```python
from build123d import *

# Parameters (mm, degrees)
SKETCH_1_W                         = 200
SKETCH_1_H                         = 27
SM_BASE_FLANGE_1_DEPTH             = 1
SM_EDGE_FLANGE_1_STRIP_W           = 7
SM_EDGE_FLANGE_1_STRIP_H           = 1
SM_EDGE_FLANGE_1_STRIP_CUT_DEPTH   = 200
SM_EDGE_FLANGE_1_STRIP_2_W         = 7
SM_EDGE_FLANGE_1_STRIP_2_H         = 1
SM_EDGE_FLANGE_1_STRIP_CUT_2_DEPTH = 200
SM_EDGE_FLANGE_1_DEPTH             = 200
SM_EDGE_FLANGE_1_BEND_DEPTH        = 200
SM_EDGE_FLANGE_2_STRIP_W           = 7
SM_EDGE_FLANGE_2_STRIP_H           = 1
SM_EDGE_FLANGE_2_STRIP_CUT_DEPTH   = 200
SM_EDGE_FLANGE_2_STRIP_2_W         = 7
SM_EDGE_FLANGE_2_STRIP_2_H         = 1
SM_EDGE_FLANGE_2_STRIP_CUT_2_DEPTH = 200
SM_EDGE_FLANGE_2_DEPTH             = 200
SM_EDGE_FLANGE_2_BEND_DEPTH        = 200
CUT_EXTRUDE_1_DEPTH                = 10
PATTERN_LINEAR_1_COUNT             = 5
PATTERN_LINEAR_1_PITCH             = 20
PATTERN_LINEAR_1_COL_COUNT         = 5
PATTERN_LINEAR_1_COL_PITCH         = 20


# Sheet-metal steps are written as plain solids
with BuildPart() as part:
    # Sketch 1 → 基体-法兰1 (new body)
    with BuildSketch(Plane.XY):
        Rectangle(SKETCH_1_W, SKETCH_1_H)
    extrude(amount=-SM_BASE_FLANGE_1_DEPTH)

    # 边线-法兰1 strip (across the edge) → 边线-法兰1 strip cut (cut)
    with BuildSketch(Plane(origin=(100, 13.5, 0), x_dir=(0, -1, 0), z_dir=(-1, 0, 0))):
        with Locations((-1, -0.5)):
            Rectangle(SM_EDGE_FLANGE_1_STRIP_W, SM_EDGE_FLANGE_1_STRIP_H)
    extrude(amount=SM_EDGE_FLANGE_1_STRIP_CUT_DEPTH, mode=Mode.SUBTRACT)

    # 边线-法兰1 strip 2 (across the edge) → 边线-法兰1 strip cut 2 (cut)
    with BuildSketch(Plane(origin=(-100, -13.5, 0), x_dir=(0, 1, 0), z_dir=(1, 0, 0))):
        with Locations((-1, -0.5)):
            Rectangle(SM_EDGE_FLANGE_1_STRIP_2_W, SM_EDGE_FLANGE_1_STRIP_2_H)
    extrude(amount=SM_EDGE_FLANGE_1_STRIP_CUT_2_DEPTH, mode=Mode.SUBTRACT)

    # 边线-法兰1 section (across the edge) → 边线-法兰1 (add)
    with BuildSketch(Plane(origin=(100, 13.5, 0), x_dir=(0, -1, 0), z_dir=(-1, 0, 0))):
        with BuildLine():
            Line((0, 1.5), (0, 6.5))
            Line((0, 6.5), (1, 6.5))
            Line((1, 6.5), (1, 1.5))
            ThreePointArc((1, 1.5), (1.439339828, 0.439339828), (2.5, 0))
            Line((2.5, 0), (2.5, -1))
            ThreePointArc((2.5, -1), (0.732233047, -0.267766953), (0, 1.5))
        make_face()
    extrude(amount=SM_EDGE_FLANGE_1_DEPTH)

    # 边线-法兰1 section 2 (across the edge) → 边线-法兰1 bend (add)
    with BuildSketch(Plane(origin=(-100, -13.5, 0), x_dir=(0, 1, 0), z_dir=(1, 0, 0))):
        with BuildLine():
            Line((0, 1.5), (0, 6.5))
            Line((0, 6.5), (1, 6.5))
            Line((1, 6.5), (1, 1.5))
            ThreePointArc((1, 1.5), (1.439339828, 0.439339828), (2.5, 0))
            Line((2.5, 0), (2.5, -1))
            ThreePointArc((2.5, -1), (0.732233047, -0.267766953), (0, 1.5))
        make_face()
    extrude(amount=SM_EDGE_FLANGE_1_BEND_DEPTH)

    # 边线-法兰2 strip (across the edge) → 边线-法兰2 strip cut (cut)
    with BuildSketch(Plane(origin=(-100, 13.5, 6.5), x_dir=(0, 0, -1), z_dir=(1, 0, 0))):
        with Locations((-1, -0.5)):
            Rectangle(SM_EDGE_FLANGE_2_STRIP_W, SM_EDGE_FLANGE_2_STRIP_H)
    extrude(amount=SM_EDGE_FLANGE_2_STRIP_CUT_DEPTH, mode=Mode.SUBTRACT)

    # 边线-法兰2 strip 2 (across the edge) → 边线-法兰2 strip cut 2 (cut)
    with BuildSketch(Plane(origin=(100, -13.5, 6.5), x_dir=(0, 0, -1), z_dir=(-1, 0, 0))):
        with Locations((-1, -0.5)):
            Rectangle(SM_EDGE_FLANGE_2_STRIP_2_W, SM_EDGE_FLANGE_2_STRIP_2_H)
    extrude(amount=SM_EDGE_FLANGE_2_STRIP_CUT_2_DEPTH, mode=Mode.SUBTRACT)

    # 边线-法兰2 section (across the edge) → 边线-法兰2 (add)
    with BuildSketch(Plane(origin=(-100, 13.5, 6.5), x_dir=(0, 0, -1), z_dir=(1, 0, 0))):
        with BuildLine():
            Line((0, 1.5), (0, 4))
            Line((0, 4), (1, 4))
            Line((1, 4), (1, 1.5))
            ThreePointArc((1, 1.5), (1.439339828, 0.439339828), (2.5, 0))
            Line((2.5, 0), (2.5, -1))
            ThreePointArc((2.5, -1), (0.732233047, -0.267766953), (0, 1.5))
        make_face()
    extrude(amount=SM_EDGE_FLANGE_2_DEPTH)

    # 边线-法兰2 section 2 (across the edge) → 边线-法兰2 bend (add)
    with BuildSketch(Plane(origin=(100, -13.5, 6.5), x_dir=(0, 0, -1), z_dir=(-1, 0, 0))):
        with BuildLine():
            Line((0, 1.5), (0, 4))
            Line((0, 4), (1, 4))
            Line((1, 4), (1, 1.5))
            ThreePointArc((1, 1.5), (1.439339828, 0.439339828), (2.5, 0))
            Line((2.5, 0), (2.5, -1))
            ThreePointArc((2.5, -1), (0.732233047, -0.267766953), (0, 1.5))
        make_face()
    extrude(amount=SM_EDGE_FLANGE_2_BEND_DEPTH)

    # 草图18 → 切除-拉伸1 (cut)
    with BuildSketch(Plane(origin=(0, 0, -1), x_dir=(-1, 0, 0), z_dir=(0, 0, -1))):
        with BuildLine():
            Line((-4, 2.25), (4, 2.25))
            ThreePointArc((4, 2.25), (6.25, 0), (4, -2.25))
            Line((4, -2.25), (-4, -2.25))
            ThreePointArc((-4, -2.25), (-6.25, 0), (-4, 2.25))
        make_face()
    cut_extrude_1 = extrude(amount=-CUT_EXTRUDE_1_DEPTH, mode=Mode.SUBTRACT)

    # 阵列(线性)1: 切除-拉伸1 ×5
    with Locations(*[(i * PATTERN_LINEAR_1_PITCH, 0, 0) for i in range(1, PATTERN_LINEAR_1_COUNT)]):
        add(cut_extrude_1, mode=Mode.SUBTRACT)

    # 阵列(线性)1 col: 切除-拉伸1 ×5
    with Locations(*[(-i * PATTERN_LINEAR_1_COL_PITCH, 0, 0) for i in range(1, PATTERN_LINEAR_1_COL_COUNT)]):
        add(cut_extrude_1, mode=Mode.SUBTRACT)


solid = part.part
```
The model under review builds one solid part; all positions refer to its coordinate system, in mm. Round coordinates to 2 decimals unless told otherwise and drop trailing zeros. Write each loop counter-clockwise with the first axis right and the second up, starting at its lowest first coordinate (ties: lowest second). Pieces come first, ordered by that corner, then holes. Notation, with made-up numbers: (34, 63) - (51, 63) arc R6 cw to (51, 73) - close; hole circle Ø3 at (70.25, 44). An arc over 180 degrees is marked (long way). Answer as CSV lines item,"result". Start each with the question number.
(1) We need section A-A on x = -61. State the section outline as (y, z) points, plus the area to 3 significant figures.
(2) To check wall thickness, follow line 1 (Y direction, x = 45, z = 1.25); line 2 (Z direction, x = -53, y = -13); line 3 (Z direction, x = 9.5, y = -15). State the ranges of each line that lie inside material, in increasing order.
(3) We need section B-B on x = 12. State the section outline as (y, z) points, plus the area to 3 significant figures.
(4) We need section D-D on y = -9. State the section outline as (x, z) points, plus the area to 3 significant figures.
(5) For pin 1 Ø0.8 at (x, z) = (3, 2) entering from +Y; pin 2 Ø0.8 at (x, z) = (-46, 2.5) entering from -Y; pin 3 Ø0.8 at (x, z) = (-81, -0.5) entering from +Y, all flat-tipped, find the tip position at first contact; note any pin that passes through.
(6) We need section C-C on y = 0. Give the number of separate pieces and of enclosed holes in the cut face, plus the area to 3 significant figures.
(7) Draft analysis for pull direction Y (two halves, no side actions). For faces 1 (the flat face through (-100, -0.1, -0.6)), 2 (the flat face through (-1, 3, 0)), state which applies: pulls with the +Y half, pulls with the -Y half, needs draft (parallel to the pull), parting line crosses it, or undercut.
Worked answers:
1,outline,"(-17.5, 5.5) - (-15, 5.5) arc R1.5 cw to (-13.5, 4) - (-13.5, 1.5) arc R2.5 ccw to (-11, -1) - (-2.25, -1) - (-2.25, 0) - (-11, 0) arc R1.5 cw to (-12.5, 1.5) - (-12.5, 4) arc R2.5 ccw to (-15, 6.5) - (-17.5, 6.5) - close; (2.25, -1) - (11, -1) arc R2.5 ccw to (13.5, 1.5) - (13.5, 4) arc R1.5 cw to (15, 5.5) - (17.5, 5.5) - (17.5, 6.5) - (15, 6.5) arc R2.5 ccw to (12.5, 4) - (12.5, 1.5) arc R1.5 cw to (11, 0) - (2.25, 0) - close"
1,area,"40.1 mm²"
2,line 1,"-13.49 to -12.48, 12.48 to 13.49"
2,line 2,"0 to 5.5"
2,line 3,"5.5 to 6.5"
3,outline,"(-17.5, 5.5) - (-15, 5.5) arc R1.5 cw to (-13.5, 4) - (-13.5, 1.5) arc R2.5 ccw to (-11, -1) - (11, -1) arc R2.5 ccw to (13.5, 1.5) - (13.5, 4) arc R1.5 cw to (15, 5.5) - (17.5, 5.5) - (17.5, 6.5) - (15, 6.5) arc R2.5 ccw to (12.5, 4) - (12.5, 1.5) arc R1.5 cw to (11, 0) - (-11, 0) arc R1.5 cw to (-12.5, 1.5) - (-12.5, 4) arc R2.5 ccw to (-15, 6.5) - (-17.5, 6.5) - close"
3,area,"44.6 mm²"
4,outline,"(-100, -1) - (100, -1) - (100, 0) - (-100, 0) - close"
4,area,"200 mm²"
5,pin 1,"y = 13.5"
5,pin 2,"y = -13.5"
5,pin 3,"y = 12.92"
6,separate pieces,"10"
6,enclosed holes,"0"
6,area,"87.5 mm²"
7,face 1,"needs draft"
7,face 2,"undercut"
